Build history of the part. All positions in model axes, mm. A direction names the side the tool comes from. Give positions to 0.01 mm unless a question says otherwise; leave off trailing zeros. Loops run counter-clockwise (first coordinate to the right, second up) from the corner with the lowest first, then second, coordinate; pieces in that order, holes last.
1) Band-saw the part on C-C on x = 36. List the corners of the cut face in (y, z).
2) Wall check: line 1 (Y direction, x = -13, z = -0.5); line 2 (Y direction, x = 12.5, z = -0.5); line 3 (X direction, y = -8.5, z = 2.75). Give the ranges that are in metal, low to high.
3) Flat gauge pins, fed straight in: P1, Ø10, axis at y = -4, z = -2.5, coming from the +X side; P2, Ø0.5, axis at y = 0, z = 3.5, coming from the +X side; P3, Ø3, axis at x = -8.5, z = 3.5, coming from the +Y side; P4, Ø5, axis at x = 9, z = 0.5, coming from the +Y side. Where does each tip first touch, or does it go through?
4) Two-plate mould, pull along X, no slides. Class faces 1 (the conical face through (41.417, -1.413, 4.486)), 2 (the flat face through (-18.5, -6.3, 0.1)), 3 (the cylindrical face through (72.605, -3.966, -0.521)): +X half, -X half, draft (parallel to the pull), parting line (faces both ways), or undercut.
5) Band-saw the part on D-D on x = 49.5. List the corners of the cut face in (y, z).
6) Band-saw the part on B-B on x = -13.5. List the corners of the cut face in (y, z), then the cut area to 3 significant figures.
7) 3-axis set-ups, long thin cutter, end or side, ignore diameter. For faces 4 (the flat face through (-15, 0, -7.5)), 5 (the flat face through (83, 0, 3)), 6 (the flat face through (-20.5, -2, 6)), 7 (the flat face through (83, 0, -3)), 8 (the cylindrical face through (51.63, -3.04, -3.32)): which of +Z, -Z, +X, -X, +Y, -Y reach the whole face in a straight line?
```python
from build123d import *

# Parameters (mm, degrees)
CHANFREIN1_SIZE              = 1
ESQUISSE2_W                  = 9.5
ESQUISSE2_H                  = 1
ENL_V_MAT_EXTRU_1_DEPTH      = 10.25
ENL_V_MAT_EXTRU_1_DEPTH_BACK = 10.25
ENL_V_MAT_EXTRU_3_DEPTH      = 10.25
ENL_V_MAT_EXTRU_3_DEPTH_BACK = 10.25


with BuildPart() as part:
    # Esquisse1 → Révolution1 (revolve)
    with BuildSketch(Plane.XY, mode=Mode.PRIVATE) as r_volution1_sk:
        with BuildLine():
            Line((-30.5, 0), (-30.5, 7))
            Line((-30.5, 7), (-20.5, 7))
            Line((-20.5, 7), (-20.5, 6))
            Line((-20.5, 6), (-18.5, 6))
            Line((-18.5, 6), (-18.5, 9.25))
            Line((-18.5, 9.25), (-2.5, 9.25))
            Line((-2.5, 9.25), (-2.5, 7.25))
            Line((-2.5, 7.25), (-1.5, 7.25))
            Line((-1.5, 7.25), (-1.5, 6.75))
            ThreePointArc((-1.5, 6.75), (-1.060660172, 5.689339828), (0, 5.25))
            Line((0, 5.25), (38.5, 5.25))
            Line((38.5, 5.25), (42.5, 4.5))
            Line((42.5, 4.5), (60.5, 4.5))
            Line((60.5, 4.5), (63.5, 4))
            Line((63.5, 4), (87.5, 4))
            Line((87.5, 4), (87.5, 0))
            Line((87.5, 0), (-30.5, 0))
        make_face()
    revolve(r_volution1_sk.sketch.rotate(Axis((-56.136256415, 0, 0), (1, 0, 0)), 90), axis=Axis((-56.136256415, 0, 0), (1, 0, 0)))  # turned: the seam where the file's is

    # Chanfrein1
    chanfrein1_edges = [part.edges().sort_by_distance(p)[0] for p in [
        (87.5, 0, -4),
        (-30.5, 0, -7),
    ]]
    chamfer(chanfrein1_edges, length=CHANFREIN1_SIZE)

    # Esquisse2 → Enlèv. mat.-Extru.1 (cut, two sides)
    with BuildSketch(Plane(origin=(0, 0, 0), x_dir=(1, 0, 0), z_dir=(0, 1, 0))) as enl_v_mat_extru_1_sk:
        with Locations((82.75, 3.5)):
            Rectangle(ESQUISSE2_W, ESQUISSE2_H)
        with Locations((82.75, -3.5)):
            Rectangle(ESQUISSE2_W, ESQUISSE2_H)
    extrude(amount=ENL_V_MAT_EXTRU_1_DEPTH, mode=Mode.SUBTRACT)
    extrude(enl_v_mat_extru_1_sk.sketch, amount=-ENL_V_MAT_EXTRU_1_DEPTH_BACK, mode=Mode.SUBTRACT)

    # Esquisse4 → Enlèv. mat.-Extru.3 (cut, two sides)
    with BuildSketch(Plane(origin=(0, 0, 0), x_dir=(1, 0, 0), z_dir=(0, 1, 0))) as enl_v_mat_extru_3_sk:
        Polygon((-10.5, 7.5), (-8.75, 9.25), (-18.5, 9.25), (-18.5, 7.5), align=None)
        Polygon((-18.5, -7.5), (-10.5, -7.5), (-8.75, -9.25), (-18.5, -9.25), align=None)
    extrude(amount=ENL_V_MAT_EXTRU_3_DEPTH, mode=Mode.SUBTRACT)
    extrude(enl_v_mat_extru_3_sk.sketch, amount=-ENL_V_MAT_EXTRU_3_DEPTH_BACK, mode=Mode.SUBTRACT)


solid = part.part
```
Findings below:
1. outline: circle Ø10.5 at (0, 0)
2. line 1: y = -9.24 to 9.24
2. line 2: y = -5.23 to 5.23
2. line 3: x = -18.5 to -2.5
3. P1: stops at x = 87.5
3. P2: stops at x = 78
3. P3: stops at y = 9.03
3. P4: stops at y = 5.25
4. face 1: +X half
4. face 2: undercut
4. face 3: draft
5. outline: circle Ø9 at (0, 0)
6. outline: (-5.41, -7.5) - (5.41, -7.5) arc R9.25 ccw to (5.41, 7.5) - (-5.41, 7.5) arc R9.25 ccw to start
6. area: 243 mm2
7. face 4: -Z, -X, +Y, -Y
7. face 5: +Z, +X, +Y, -Y
7. face 6: none
7. face 7: -Z, +X, +Y, -Y
7. face 8: +X
